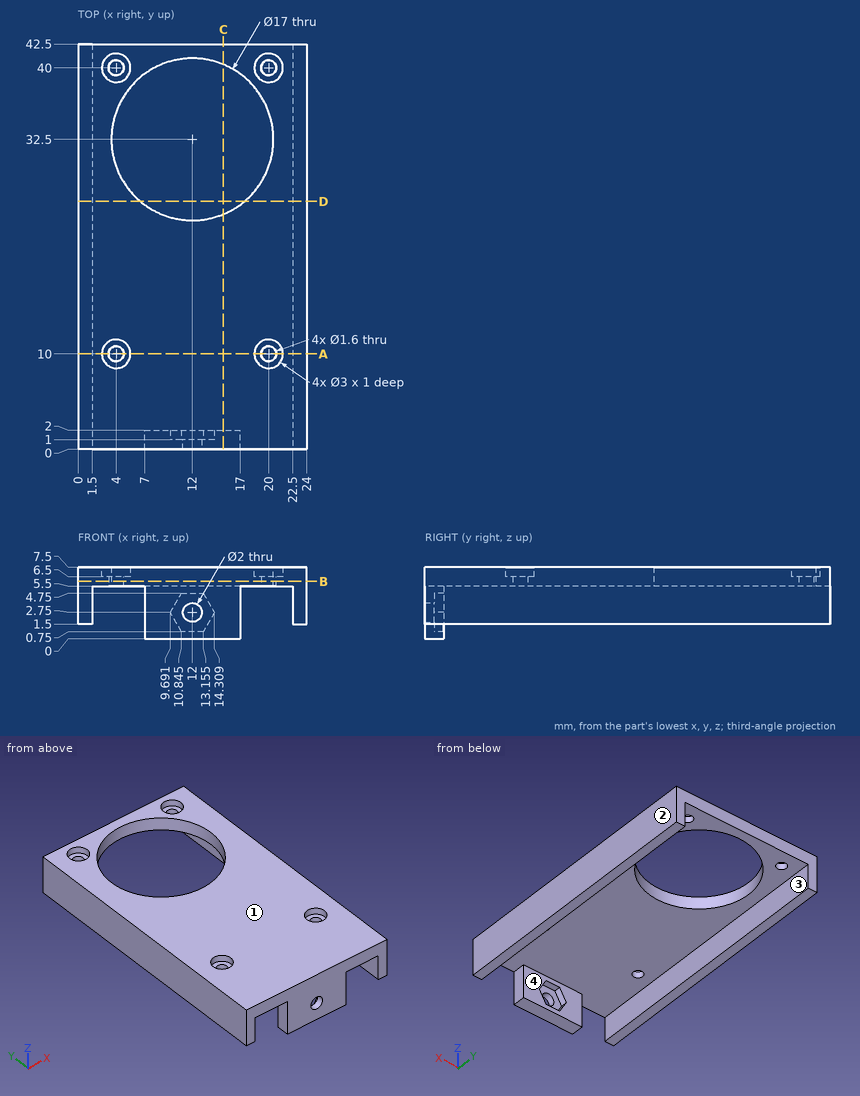
Answer from the drawing. Dimensions are ordinates in mm from the lowest x, y and z of the part. Give positions to 0.01 mm unless a question says otherwise; leave off trailing zeros. Order: outer loops, then holes, each group sorted by start corner. A loop starts at its lowest first (then second) coordinate and runs counter-clockwise, first axis right, second up. Notation, with made-up numbers: (-22.5, -27) - (-8.5, -27) arc R20 cw to (-8.5, -9) - close; hole circle Ø11 at (-16.75, 59.25). An arc over 180 degrees is marked (long way). Use one line per item in the form item = value.
1) Find section D-D on y = 26. Determine the outline of the cut face in (x, z), and give its area (3 significant figures).
Verdict:
outline = (0, 1.5) - (1.5, 1.5) - (1.5, 5.5) - (6.52, 5.5) - (6.52, 7.5) - (0, 7.5) - close; (17.48, 5.5) - (22.5, 5.5) - (22.5, 1.5) - (24, 1.5) - (24, 7.5) - (17.48, 7.5) - close
area = 38.1 mm^2
2) Find section B-B on z = 6. Determine the outline of the cut face in (x, y), and give its area (3 significant figures).
Verdict:
outline = (0, 0) - (24, 0) - (24, 42.5) - (0, 42.5) - close; hole circle Ø1.6 at (4, 10); hole circle Ø1.6 at (4, 40); hole circle Ø17 at (12, 32.5); hole circle Ø1.6 at (20, 10); hole circle Ø1.6 at (20, 40)
area = 785 mm^2
3) The mould has two halves that part along X. Classify the marked faces 1, 2, 3 and 4: released by +X, released by -X, zero draft, split by the parting line, or undercut.
Verdict:
face_1 = zero draft
face_2 = released by +X
face_3 = undercut
face_4 = undercut
4) Find section A-A on y = 10. Determine the outline of the cut face in (x, z).
Verdict:
outline = (0, 1.5) - (1.5, 1.5) - (1.5, 5.5) - (3.2, 5.5) - (3.2, 6.5) - (2.5, 6.5) - (2.5, 7.5) - (0, 7.5) - close; (4.8, 5.5) - (19.2, 5.5) - (19.2, 6.5) - (18.5, 6.5) - (18.5, 7.5) - (5.5, 7.5) - (5.5, 6.5) - (4.8, 6.5) - close; (20.8, 5.5) - (22.5, 5.5) - (22.5, 1.5) - (24, 1.5) - (24, 7.5) - (21.5, 7.5) - (21.5, 6.5) - (20.8, 6.5) - close
5) Find section C-C on x = 15.25. Determine the outline of the cut face in (y, z).
Verdict:
outline = (0, 0) - (2, 0) - (2, 5.5) - (24.65, 5.5) - (24.65, 7.5) - (0, 7.5) - close; (40.35, 5.5) - (42.5, 5.5) - (42.5, 7.5) - (40.35, 7.5) - close
6) Consider probe 1 along X at (y, z) = (10, 5.8); probe 2 along X at (y, z) = (22, 4); probe 3 along Z at (x, y) = (12, 0.65). Determine where each line is inside the solid, lowest interval first. Write a range as [from, to].
Verdict:
probe_1 = [0, 3.2], [4.8, 19.2], [20.8, 24]
probe_2 = [0, 1.5], [22.5, 24]
probe_3 = [0, 1.75], [3.75, 7.5]
7) Each of these flat-tipped pins is pushed along its axis until it touches: pin 1 (8 mm diameter, centred on x = 8, y = 32, fed in from +Z); pin 2 (3 mm diameter, centred on x = 11, z = 4.5, fed in from -Y); pin 3 (1.6 mm diameter, centred on x = 11.5, z = 2, fed in from +Y); pin 4 (12 mm diameter, centred on x = 12.5, y = 24, fed in from -Z). Where does it stop, or does it pass through?
Verdict:
pin_1 = through
pin_2 = 0
pin_3 = 1
pin_4 = 5.5
